from build123d import *

# Parameters (mm, degrees)
IZIM1_W                          = 20
IZIM1_H                          = 5
Y_KSEKLIK_EKSTR_ZYON3_DEPTH      = 70
IZIM2_R                          = 1
IZIM2_W                          = 13
IZIM2_H                          = 23
KES_EKSTR_ZYON1_DEPTH            = 70
Y_KSEKLIK_EKSTR_ZYON4_DEPTH      = 20
Y_KSEKLIK_EKSTR_ZYON4_DEPTH_BACK = 25
IZIM3_W                          = 20
IZIM3_H                          = 5
IZIM4_R                          = 1.75
KES_EKSTR_ZYON2_DEPTH            = 25


with BuildPart() as part:
    # Çizim1 → Yükseklik-Ekstrüzyon3 (new body)
    with BuildSketch(Plane(origin=(0, 0, 0), x_dir=(1, 0, 0), z_dir=(0, 1, 0))):
        with Locations((10, 2.5)):
            Rectangle(IZIM1_W, IZIM1_H)
    extrude(amount=Y_KSEKLIK_EKSTR_ZYON3_DEPTH)

    # Çizim2 → Kes-Ekstrüzyon1 (cut)
    with BuildSketch(Plane.XY):
        with Locations((10, 67.5)):
            Circle(IZIM2_R)
        with Locations((10, 39.5)):
            Circle(IZIM2_R)
        with Locations((10, 53.5)):
            Rectangle(IZIM2_W, IZIM2_H)
    extrude(amount=-KES_EKSTR_ZYON1_DEPTH, mode=Mode.SUBTRACT)

    # Çizim3 → Yükseklik-Ekstrüzyon4 (add, two sides: drawn at the far end of the back side and taken through both)
    with BuildSketch(Plane.XY.offset(-Y_KSEKLIK_EKSTR_ZYON4_DEPTH_BACK)):
        with Locations((10, 2.5)):
            Rectangle(IZIM3_W, IZIM3_H)
    extrude(amount=Y_KSEKLIK_EKSTR_ZYON4_DEPTH + Y_KSEKLIK_EKSTR_ZYON4_DEPTH_BACK)

    # Çizim4 → Kes-Ekstrüzyon2 (cut)
    with BuildSketch(Plane(origin=(0, 5, 0), x_dir=(1, 0, 0), z_dir=(0, 1, 0))):
        with Locations(Location((10, -15, 0), (0, 0, 270))):
            Circle(IZIM4_R)
        with Locations(Location((10, 20, 0), (0, 0, 270))):
            Circle(IZIM4_R)
    extrude(amount=-KES_EKSTR_ZYON2_DEPTH, mode=Mode.SUBTRACT)


solid = part.part
Can you work these out from the model? Positions are in its coordinate system, mm. A direction names the side the tool comes from. Give positions to 0.01 mm unless a question says otherwise; leave off trailing zeros. Loops run counter-clockwise (first coordinate to the right, second up) from the corner with the lowest first, then second, coordinate; pieces in that order, holes last. Notation, with made-up numbers: (-0.5, -38.75) -> (3.5, -38.75) arc R24 cw to (3.5, -21.75) -> close; hole circle Ø1 at (28, -27.75). An arc over 180 degrees is marked (long way). Return JSON: item names as keys, results as strings.
Q1. For pin 1 Ø6 at (x, y) = (10, 35) entering from -Z; pin 2 Ø3 at (x, y) = (2, 33.5) entering from +Z; pin 3 Ø3 at (x, z) = (10, -20) entering from -Y; pin 4 Ø1.5 at (x, z) = (5.5, 14) entering from +Y, each with a flat end and sliding along its axis, tell me the tip position at first contact or that it passes through.
Checks:
{"pin 1": "stops at z = -5", "pin 2": "stops at z = 0", "pin 3": "passes through", "pin 4": "stops at y = 5"}
Q2. I want a section at B-B, the plane y = 55.5. List the corners of the cut face in (x, z) for me, then the cut area to 3 significant figures.
Checks:
{"outline": "(0, -5) -> (3.5, -5) -> (3.5, 0) -> (0, 0) -> close; (16.5, -5) -> (20, -5) -> (20, 0) -> (16.5, 0) -> close", "area": "35.0 mm2"}
Q3. I want a section at C-C, the plane z = -20. List the corners of the cut face in (x, y) for me.
Checks:
{"outline": "(0, 0) -> (8.25, 0) -> (8.25, 5) -> (0, 5) -> close; (11.75, 0) -> (20, 0) -> (20, 5) -> (11.75, 5) -> close"}
Q4. We'd pull the mould along Z, two halves only. Please class faces 1 (the face through (10, 70, -3)), 2 (the face through (10, 3, -25)), 3 (the face through (11.18, 2.54, -21.29)): released by +Z, released by -Z, zero draft, split by the parting line, or undercut.
Checks:
{"face 1": "zero draft", "face 2": "released by -Z", "face 3": "undercut"}
Q5. On a 3-axis mill with a long thin cutter (end or side, diameter ignored), from which of +Z, -Z, +X, -X, +Y, -Y can I reach the whole of each face in a straight line? I mean faces 4 (the face through (10, 5, -15)), 5 (the face through (20, 22, -3)), 6 (the face through (16.5, 53, -2)), 7 (the face through (10, 5, 10)). Say none if no direction works.
Checks:
{"face 4": "-Z, +X, -X, +Y", "face 5": "+Z, -Z, +X, +Y, -Y", "face 6": "+Z, -Z", "face 7": "+Z, +X, -X, +Y"}
Q6. I want a section at A-A, the plane x = 13. List the corners of the cut face in (y, z) for me.
Checks:
{"outline": "(0, -25) -> (5, -25) -> (5, -5) -> (42, -5) -> (42, 0) -> (5, 0) -> (5, 20) -> (0, 20) -> close; (65, -5) -> (70, -5) -> (70, 0) -> (65, 0) -> close"}
Q7. I need wall thicknesses on probe 1 along Y at (x, z) = (10, -1.65); probe 2 along X at (y, z) = (67.5, -2.4); probe 3 along X at (y, z) = (3, 15). Which ranges of each line are inside material? Lowest first, please.
Checks:
{"probe 1": "y = 0 to 38.5, 40.5 to 42, 65 to 66.5, 68.5 to 70", "probe 2": "x = 0 to 9, 11 to 20", "probe 3": "x = 0 to 8.25, 11.75 to 20"}
Q8. I want a section at D-D, the plane x = 10. List the corners of the cut face in (y, z) for me.
Checks:
{"outline": "(0, -25) -> (5, -25) -> (5, -21.75) -> (0, -21.75) -> close; (0, -18.25) -> (5, -18.25) -> (5, -5) -> (38.5, -5) -> (38.5, 0) -> (5, 0) -> (5, 13.25) -> (0, 13.25) -> close; (0, 16.75) -> (5, 16.75) -> (5, 20) -> (0, 20) -> close; (40.5, -5) -> (42, -5) -> (42, 0) -> (40.5, 0) -> close; (65, -5) -> (66.5, -5) -> (66.5, 0) -> (65, 0) -> close; (68.5, -5) -> (70, -5) -> (70, 0) -> (68.5, 0) -> close"}
